from build123d import *

# Parameters (mm, degrees)
F3_COPIES_COUNT = 4


# Not quite as in the source:
# - a pattern or mirror of a feature is missing from the dataset's text; its kind, count and spacing are read off the source's solid


with BuildPart() as f1:
    # F0 (on Right) → F1 (revolve)
    with BuildSketch(Plane.YZ):
        with BuildLine():
            Line((5.1, 2), (5.1, 0))
            Line((5.1, 0), (8.2, 0))
            ThreePointArc((8.2, 0), (7.6142135624, 1.4142135624), (6.2, 2))
            Line((6.2, 2), (5.1, 2))
        make_face()
    revolve(axis=Axis((0, 0, 1), (0, 0, 1)))

    # F2 (on Right) → F3 (revolve, cut)
    with BuildSketch(Plane.YZ):
        Polygon((-6.45, 0.5), (-6.7, 0.5), (-6.7, 0), (-5.7, 0), (-6.2, 1), align=None)
    f3 = revolve(axis=Axis((0, -6.7, 0.25), (0, 0, 1)), mode=Mode.SUBTRACT)

    # F3_copies: F3 ×4 about axis
    f3_copies_axis = Axis((0, 0, 0), (0, 0, 1))
    for i in range(1, F3_COPIES_COUNT):
        add(f3.rotate(f3_copies_axis, i * 360 / F3_COPIES_COUNT), mode=Mode.SUBTRACT)


solid = f1.part
Input: part model. Units: mm. Frame: model coordinates. Coordinates: 2 decimals unless noted, no trailing zeros. Order: outer loops, then holes, each group sorted by start corner. A loop starts at its lowest first (then second) coordinate and runs counter-clockwise, first axis right, second up. Notation, with made-up numbers: M -34.5,2.25 L 18.5,2.25 A24 cw 18.5,25.25 Z; hole C 27.5,-20.75 d11. An arc over 180 degrees is marked long. One line per question, with ' | ' between items.
Item 1: Section C-C (z = 1.2). Output: boundary loops of the cut face in (x, y).
Geometry results:
outline: C 0,0 d15.6; hole C 0,0 d10.2
Item 2: Section A-A (y = 0). Output: boundary loops of the cut face in (x, z).
Geometry results:
outline: M -8.2,0 L -7.7,0 L -7.2,1 L -6.95,0.5 L -6.45,0.5 L -6.2,1 L -5.7,0 L -5.1,0 L -5.1,2 L -6.2,2 A2 ccw Z; M 5.1,0 L 5.7,0 L 6.2,1 L 6.45,0.5 L 6.95,0.5 L 7.2,1 L 7.7,0 L 8.2,0 A2 ccw 6.2,2 L 5.1,2 Z
Item 3: Draft query along X for faces 1 (the cylindrical face through (4.5, 2.4, 1)), 2 (the flat face through (4, 4, 0)). Return one class per face: released by +X, released by -X, zero draft, split by the parting line, or undercut.
Geometry results:
face 1: undercut | face 2: zero draft
Item 4: Ray query, line 1 along Y through (x, z) = (-3.75, 1.3); line 2 along Y through (x, z) = (-0.25, 1.05); line 3 along X through (y, z) = (0, 1.65). Return the intervals inside material, ascending.
Geometry results:
line 1: y = -6.75 to -3.46, 3.46 to 6.75 | line 2: y = -7.9 to -5.09, 5.09 to 7.9 | line 3: x = -7.33 to -5.1, 5.1 to 7.33
Item 5: Pin query (flat end, axial travel): pin 1 (0.6 mm diameter, centred on x = 0, y = -6.5, fed in from -Z); pin 2 (9 mm diameter, centred on x = 0, y = 0, fed in from -Z); pin 3 (1 mm diameter, centred on y = -3, z = 0.5, fed in from +X). Return the tip coordinate at first contact, or that it passes through.
Geometry results:
pin 1: stops at z = 0.5 | pin 2: passes through | pin 3: stops at x = 7.77
